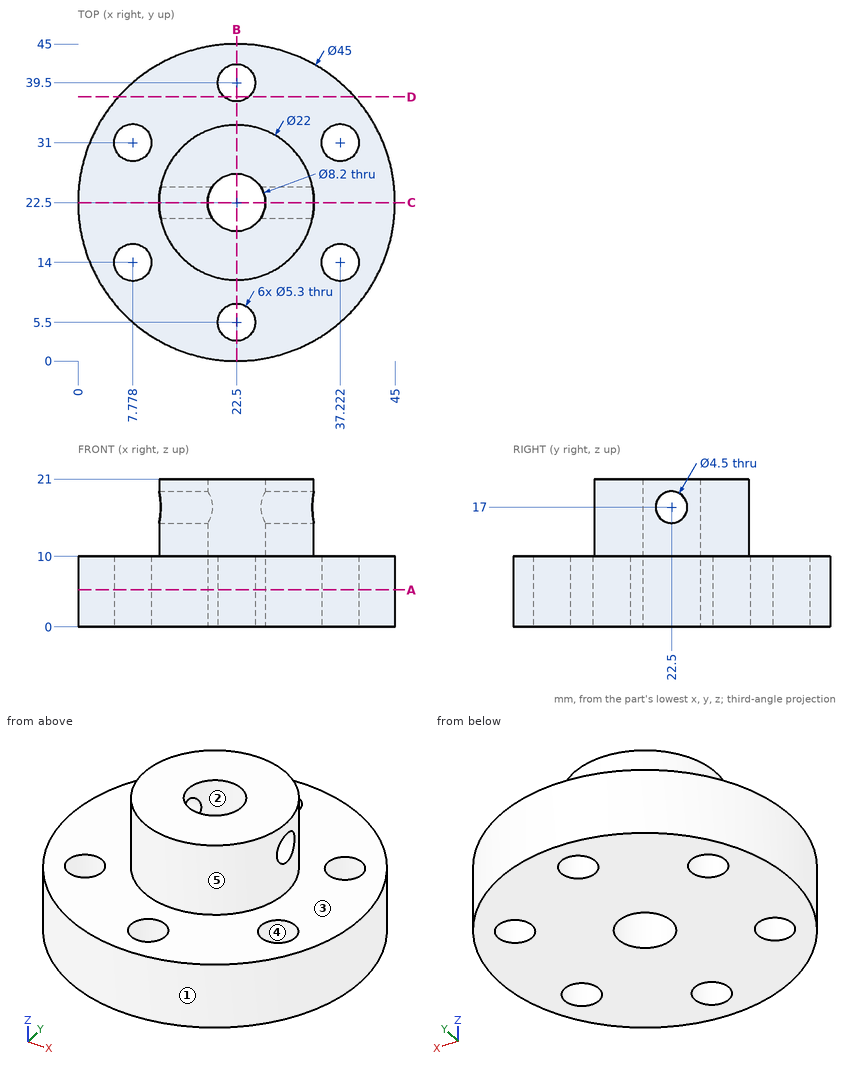
Answer from the drawing. Dimensions are ordinates in mm from the lowest x, y and z of the part. A direction names the side the tool comes from. Round coordinates to 2 decimals unless told otherwise and drop trailing zeros. Write each loop counter-clockwise with the first axis right and the second up, starting at its lowest first coordinate (ties: lowest second). Pieces come first, ordered by that corner, then holes.
1. The part is cut by section D-D, the plane y = 37.5. Determine the outline of the cut face in (x, z).
2. Straight lines are drawn through the part: L1, parallel to Z at x = 30.25, y = 22.5; L2, parallel to Y at x = 36, z = 5.5; L3, parallel to Y at x = 22.5, z = 8.25. For each, find the intervals that lie inside material, in ascending order.
3. Which of the six approach directions +Z, -Z, +X, -X, +Y, -Y give full straight-line access (tool end or side, diameter ignored) to the marked faces 4 and 5?
4. Given pin 1 Ø1.5 at (x, y) = (37, 6) entering from +Z; pin 2 Ø6 at (y, z) = (31.5, 8.5) entering from -X (1 decimal); pin 3 Ø5 at (x, y) = (7.78, 31) entering from +Z; pin 4 Ø4 at (y, z) = (28.5, 6.5) entering from +X, each flat-ended and moving along its own axis, determine where each tip first touches the part or whether it passes through.
5. The part is cut by section B-B, the plane x = 22.5. Determine the outline of the cut face in (y, z).
6. The part is cut by section C-C, the plane y = 22.5. Determine the outline of the cut face in (x, z), then the cut area to 3 significant figures.
7. The part is cut by section A-A, the plane z = 5.25. Determine the outline of the cut face in (x, y).
8. Determine the mould class of the marked faces 1, 2 and 3 for opening direction X: pulls with the +X half, pulls with the -X half, needs draft (parallel to the pull), parting line crosses it, or undercut.
Values:
1. outline: (5.73, 0) - (20.76, 0) - (20.76, 10) - (5.73, 10) - close; (24.24, 0) - (39.27, 0) - (39.27, 10) - (24.24, 10) - close
2. L1: z = 0 to 14.75, 19.25 to 21
2. L2: y = 4.5 to 11.65, 16.35 to 28.65, 33.35 to 40.5
2. L3: y = 0 to 2.85, 8.15 to 18.4, 26.6 to 36.85, 42.15 to 45
3. face 4: +Z, -Z
3. face 5: +Z
4. pin 1: stops at z = 10
4. pin 2: stops at x = 0.8
4. pin 3: passes through
4. pin 4: stops at x = 44.64
5. outline: (0, 0) - (2.85, 0) - (2.85, 10) - (0, 10) - close; (8.15, 0) - (18.4, 0) - (18.4, 21) - (11.5, 21) - (11.5, 10) - (8.15, 10) - close; (26.6, 0) - (36.85, 0) - (36.85, 10) - (33.5, 10) - (33.5, 21) - (26.6, 21) - close; (42.15, 0) - (45, 0) - (45, 10) - (42.15, 10) - close
6. outline: (0, 0) - (18.4, 0) - (18.4, 14.75) - (11.5, 14.75) - (11.5, 10) - (0, 10) - close; (11.5, 19.25) - (18.4, 19.25) - (18.4, 21) - (11.5, 21) - close; (26.6, 0) - (45, 0) - (45, 10) - (33.5, 10) - (33.5, 14.75) - (26.6, 14.75) - close; (26.6, 19.25) - (33.5, 19.25) - (33.5, 21) - (26.6, 21) - close
6. area: 458 mm2
7. outline: circle Ø45 at (22.5, 22.5); hole circle Ø5.3 at (7.78, 14); hole circle Ø5.3 at (7.78, 31); hole circle Ø8.2 at (22.5, 22.5); hole circle Ø5.3 at (22.5, 5.5); hole circle Ø5.3 at (22.5, 39.5); hole circle Ø5.3 at (37.22, 14); hole circle Ø5.3 at (37.22, 31)
8. face 1: parting line crosses it
8. face 2: undercut
8. face 3: needs draft
